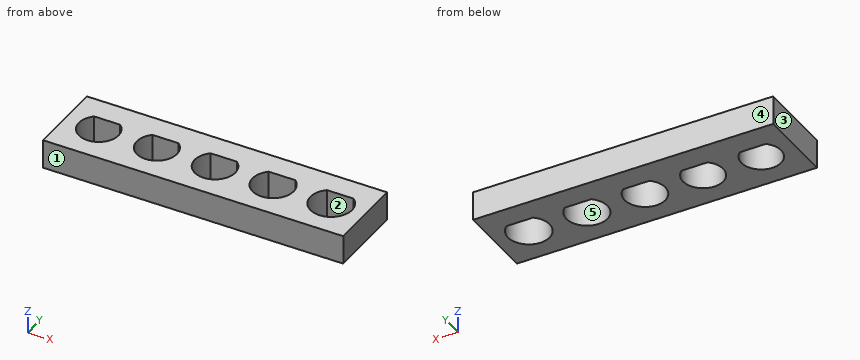
```python
from build123d import *

# Parameters (mm, degrees)
SKETCH1_W           = 31
SKETCH1_H           = 8
BOSS_EXTRUDE1_DEPTH = 3


with BuildPart() as part:
    # Sketch1 → Boss-Extrude1 (new body)
    with BuildSketch(Plane.XY):
        with Locations((15.5, 4)):
            Rectangle(SKETCH1_W, SKETCH1_H)
        with BuildLine():
            Line((2.158359214, 5.55), (4.841640786, 5.55))
            ThreePointArc((4.841640786, 5.55), (3.5, 1.95), (2.158359214, 5.55))
        make_face(mode=Mode.SUBTRACT)
        with BuildLine():
            Line((8.149074391, 5.575), (10.850925609, 5.575))
            ThreePointArc((10.850925609, 5.575), (9.5, 1.925), (8.149074391, 5.575))
        make_face(mode=Mode.SUBTRACT)
        with BuildLine():
            Line((14.139852949, 5.6), (16.860147051, 5.6))
            ThreePointArc((16.860147051, 5.6), (15.5, 1.9), (14.139852949, 5.6))
        make_face(mode=Mode.SUBTRACT)
        with BuildLine():
            Line((20.130693606, 5.625), (22.869306394, 5.625))
            ThreePointArc((22.869306394, 5.625), (21.5, 1.875), (20.130693606, 5.625))
        make_face(mode=Mode.SUBTRACT)
        with BuildLine():
            Line((26.121595125, 5.65), (28.878404875, 5.65))
            ThreePointArc((28.878404875, 5.65), (27.5, 1.85), (26.121595125, 5.65))
        make_face(mode=Mode.SUBTRACT)
    extrude(amount=BOSS_EXTRUDE1_DEPTH)


solid = part.part
```
Input: part model. Units: mm. Frame: model coordinates. Face numbers are marked on the shaded views. A direction names the side the tool comes from. Coordinates: 2 decimals unless noted, no trailing zeros. Loops run counter-clockwise (first coordinate to the right, second up) from the corner with the lowest first, then second, coordinate; pieces in that order, holes last.
Q1. Line query: line 1 along X through (y, z) = (4, 1.7) (3 decimals); line 2 along Y through (x, z) = (3.5, 2.05); line 3 along Y through (x, z) = (21.5, 0.85) (3 decimals). Output: solid intervals per line, ascending.
Results are:
line 1: x = 0 to 1.45, 5.55 to 7.425, 11.575 to 13.4, 17.6 to 19.375, 23.625 to 25.35, 29.65 to 31
line 2: y = 0 to 1.95, 5.55 to 8
line 3: y = 0 to 1.875, 5.625 to 8
Q2. Section C-C, the plane z = 2.3. Return the cut outline in (x, y) (3 decimals), and give its area (3 significant figures).
Results are:
outline: (0, 0) - (31, 0) - (31, 8) - (0, 8) - close; hole (2.158, 5.55) arc R2.05 ccw (long way) to (4.842, 5.55) - close; hole (8.149, 5.575) arc R2.075 ccw (long way) to (10.851, 5.575) - close; hole (14.14, 5.6) arc R2.1 ccw (long way) to (16.86, 5.6) - close; hole (20.131, 5.625) arc R2.125 ccw (long way) to (22.869, 5.625) - close; hole (26.122, 5.65) arc R2.15 ccw (long way) to (28.878, 5.65) - close
area: 183 mm2
Q3. Section D-D, the plane x = 15.5. Return the cut outline in (y, z).
Results are:
outline: (0, 0) - (1.9, 0) - (1.9, 3) - (0, 3) - close; (5.6, 0) - (8, 0) - (8, 3) - (5.6, 3) - close
Q4. Section A-A, the plane x = 9.5. Return the cut outline in (y, z) (3 decimals).
Results are:
outline: (0, 0) - (1.925, 0) - (1.925, 3) - (0, 3) - close; (5.575, 0) - (8, 0) - (8, 3) - (5.575, 3) - close
Q5. Mould query, pull axis Y, two halves, no side actions, for the marked faces 3, 4 and 5. Classes: +Y half, -Y half, draft (parallel to the pull), parting line (faces both ways), or undercut.
Results are:
face 3: draft
face 4: +Y half
face 5: undercut
Q6. Section B-B, the plane y = 4. Return the cut outline in (x, z) (3 decimals), and give its area (3 significant figures).
Results are:
outline: (0, 0) - (1.45, 0) - (1.45, 3) - (0, 3) - close; (5.55, 0) - (7.425, 0) - (7.425, 3) - (5.55, 3) - close; (11.575, 0) - (13.4, 0) - (13.4, 3) - (11.575, 3) - close; (17.6, 0) - (19.375, 0) - (19.375, 3) - (17.6, 3) - close; (23.625, 0) - (25.35, 0) - (25.35, 3) - (23.625, 3) - close; (29.65, 0) - (31, 0) - (31, 3) - (29.65, 3) - close
area: 30.0 mm2
Q7. Set-up query: the marked faces 1 and 2. Return all of +Z, -Z, +X, -X, +Y, -Y with unobstructed straight access to the full face (end or side cutting, diameter ignored); none if empty.
Results are:
face 1: +Z, -Z, +X, -X, -Y
face 2: +Z, -Z
